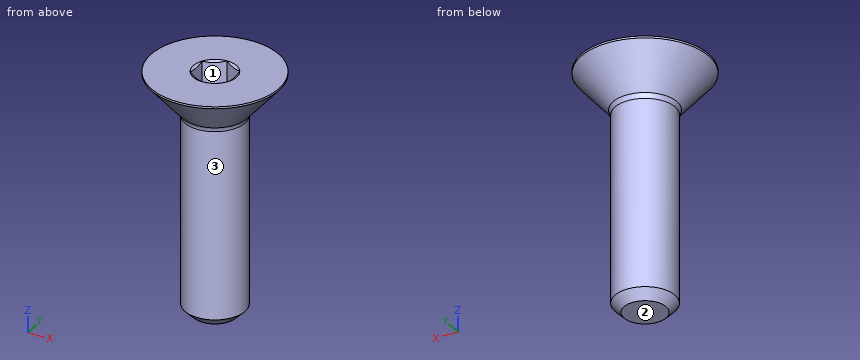
from build123d import *

# Parameters (mm, degrees)
SKETCH1_W          = 25.4
SKETCH1_H          = 3.175
CHAMFER1_SIZE      = 0.9525
CUT_EXTRUDE2_DEPTH = 2.86258


with BuildPart() as part:
    # Sketch1 → Revolve1 (revolve)
    with BuildSketch(Plane(origin=(0, 0, 0), x_dir=(0, 0, -1), z_dir=(1, 0, 0))):
        with Locations((12.7, 1.5875)):
            Rectangle(SKETCH1_W, SKETCH1_H)
    revolve(axis=Axis((0, 0, -25.4), (0, 0, 1)))

    # Chamfer1
    chamfer1_edges = [part.edges().sort_by_distance(p)[0] for p in [
        (0, -3.175, -25.4),
    ]]
    chamfer(chamfer1_edges, length=CHAMFER1_SIZE)

    # Sketch7 → Revolve2 (revolve)
    with BuildSketch(Plane(origin=(0, 0, 0), x_dir=(0, 0, -1), z_dir=(1, 0, 0)), mode=Mode.PRIVATE) as revolve2_sk:
        with BuildLine():
            Line((0, 6.7437), (0.20447, 6.7437))
            Line((0.20447, 6.7437), (4.0894, 3.366581874))
            ThreePointArc((4.0894, 3.366581874), (4.328282675, 3.224461616), (4.601808997, 3.175))
            Line((4.601808997, 3.175), (4.601808997, 0))
            Line((4.601808997, 0), (0, 0))
            Line((0, 0), (0, 6.7437))
        make_face()
    revolve(revolve2_sk.sketch.rotate(Axis((0, 0, 0), (0, 0, -1)), 180), axis=Axis((0, 0, 0), (0, 0, -1)))

    # Boss-Extrude1 cone 1 section (through the dimple's axis) → Boss-Extrude1 (revolve)
    with BuildSketch(Plane(origin=(0, 0, -4.601808997), x_dir=(0, -1, 0), z_dir=(1, 0, 0))):
        Polygon((0, 0), (3.175, 0), (0, 3.06606186), align=None)
    revolve(axis=Axis((0, 0, -4.601808997), (0, 0, -1)))

    # Sketch5 → Cut-Extrude2 (cut)
    with BuildSketch(Plane.XY):
        Polygon((0, 2.291358881), (-1.984375, 1.14567944), (-1.984375, -1.14567944), (0, -2.291358881), (1.984375, -1.14567944), (1.984375, 1.14567944), align=None)
    extrude(amount=-CUT_EXTRUDE2_DEPTH, mode=Mode.SUBTRACT)

    # Cut-Extrude3 cone 1 section (through the dimple's axis) → Cut-Extrude3 (revolve, cut)
    with BuildSketch(Plane(origin=(0, 0, 0), x_dir=(0, -1, 0), z_dir=(1, 0, 0))):
        Polygon((0, 0), (2.291358881, 0), (0, 1.322916667), align=None)
    revolve(axis=Axis((0, 0, 0), (0, 0, -1)), mode=Mode.SUBTRACT)


solid = part.part
Geometry check sheet. Reference: the model listing, model coordinates, mm. Face numbers are marked on the shaded views. Give positions to 0.01 mm unless a question says otherwise; leave off trailing zeros. Loops run counter-clockwise (first coordinate to the right, second up) from the corner with the lowest first, then second, coordinate; pieces in that order, holes last. Notation, with made-up numbers: M -11.5,71 L -6.5,71 A26 cw -6.5,101 Z; hole C 5,45 d7. An arc over 180 degrees is marked long. Answer as a JSON object with one key per item and string values. Group by question number.
Item 1: Sectioned sample at B-B on z = -16. Record the boundary of the cut face in (x, y) (3 decimals).
Item 2: Material ranges on L1, parallel to Z at x = -0.5, y = 1; L2, parallel to Z at x = -4, y = 0.25; L3, parallel to X at y = 2.25, z = -8.5, recorded low to high.
Item 3: Gauge pin test, flat ends, axial feed: pin 1 (1.1 mm diameter, centred on y = -0.5, z = -1, fed in from -X); pin 2 (1.1 mm diameter, centred on y = 0, z = -1.5, fed in from +X); pin 3 (1 mm diameter, centred on y = -4, z = -13, fed in from +X); pin 4 (6 mm diameter, centred on y = 5, z = -9, fed in from -X). Record the tip position at first contact, or that the pin passes through.
Item 4: Mould release check, pull along Y, two halves, no side actions. Record for the marked faces 1, 2 and 3: pulls with the +Y half, pulls with the -Y half, needs draft (parallel to the pull), parting line crosses it, or undercut.
Findings below:
{
 "1": {"outline": "C 0,0 d6.35"},
 "2": {"L1": "-25.4 to -2.86", "L2": "-3.35 to 0", "L3": "-2.24 to 2.24"},
 "3": {"pin 1": "x = -6.51", "pin 2": "x = 6.1", "pin 3": "through", "pin 4": "x = -2.47"},
 "4": {"face 1": "undercut", "face 2": "needs draft", "face 3": "parting line crosses it"}
}
